Input: part model. Units: mm. Frame: model coordinates. Give positions to 0.01 mm unless a question says otherwise; leave off trailing zeros. Order: outer loops, then holes, each group sorted by start corner. A loop starts at its lowest first (then second) coordinate and runs counter-clockwise, first axis right, second up. Notation, with made-up numbers: M 19,60 L 61,60 A19 ccw 61,94 Z; hole C 49,-4 d8. An arc over 180 degrees is marked long. Use a Markdown table: item, result.
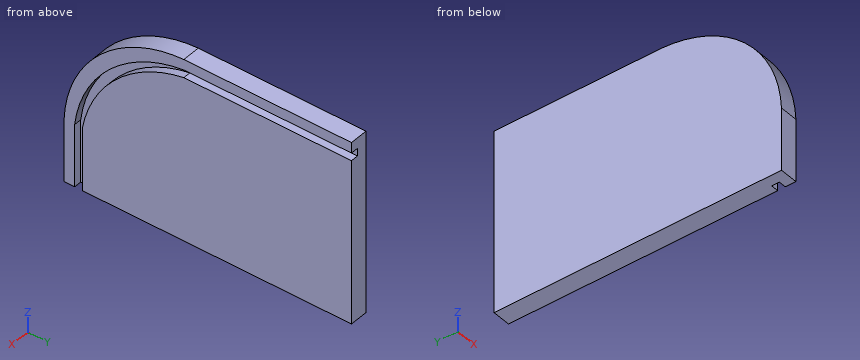
from build123d import *

# Parameters (mm, degrees)
F1_DEPTH = 19
F3_DEPTH = 8


with BuildPart() as f1:
    # F0 (on Right) → F1 (new body)
    with BuildSketch(Plane.YZ):
        with BuildLine():
            Line((150, 95), (-25, 95))
            ThreePointArc((-25, 95), (-111.955644, 57.084235), (-150, -29.815225))
            Line((-150, -29.815225), (-150, -40))
            Line((-150, -40), (-150, -95))
            Line((-150, -95), (150, -95))
            Line((150, -95), (150, 95))
        make_face()
    extrude(amount=F1_DEPTH)

    # F2 (on face) → F3 (cut)
    with BuildSketch(Plane.YZ.offset(19)):
        with BuildLine():
            Line((150, 76), (150, 84))
            Line((150, 84), (-25, 84))
            ThreePointArc((-25, 84), (-101.75341, 46.877867), (-139, -29.815225))
            Line((-139, -29.815225), (-139, -95))
            Line((-139, -95), (-131, -95))
            Line((-131, -95), (-131, -29.815225))
            ThreePointArc((-131, -29.815225), (-94.770081, 39.891752), (-25, 76))
            Line((-25, 76), (150, 76))
        make_face()
    extrude(amount=-F3_DEPTH, mode=Mode.SUBTRACT)


solid = f1.part
1) Cut plane B-B on y = -87.5. Return loops of the section in (x, z), and give its area (3 significant figures).
Response values:
| item | result |
|---|---|
| outline | M 0,-95 L 19,-95 L 19,46.62 L 11,46.62 L 11,59.18 L 19,59.18 L 19,76.26 L 0,76.26 Z |
| area | 3,150 mm² |
2) First-contact query: pin 1 Ø1.5 at (x, z) = (9, -13) entering from -Y; pin 2 Ø4 at (y, z) = (-18, -28.5) entering from -X; pin 3 Ø3 at (x, z) = (7, 51.5) entering from -Y; pin 4 Ø6 at (x, z) = (4, 42.5) entering from -Y. Flat tips, straight axial feed; report the tip coordinate or a pass-through.
Response values:
| item | result |
|---|---|
| pin 1 | stops at y = -148.37 |
| pin 2 | stops at x = 0 |
| pin 3 | stops at y = -118.54 |
| pin 4 | stops at y = -126.7 |
3) Cut plane A-A on x = 6.5. Return loops of the section in (y, z).
Response values:
| item | result |
|---|---|
| outline | M -150,-95 L 150,-95 L 150,95 L -25,95 A130 ccw -150,-29.82 Z |
4) Cut plane C-C on z = 27. Return loops of the section in (x, y), and give its area (3 significant figures).
Response values:
| item | result |
|---|---|
| outline | M 0,-134.41 L 19,-134.41 L 19,-118.06 L 11,-118.06 L 11,-106.08 L 19,-106.08 L 19,150 L 0,150 Z |
| area | 5,310 mm² |
5) Material intervals for line 1 (Y direction, x = 17, z = -84); line 2 (Z direction, x = 15.5, y = 49.5); line 3 (X direction, y = -105.5, z = 28), sorted ascending. Write a range as from..to.
Response values:
| item | result |
|---|---|
| line 1 | y = -150..-139, -131..150 |
| line 2 | z = -95..76, 84..95 |
| line 3 | x = 0..11 |
